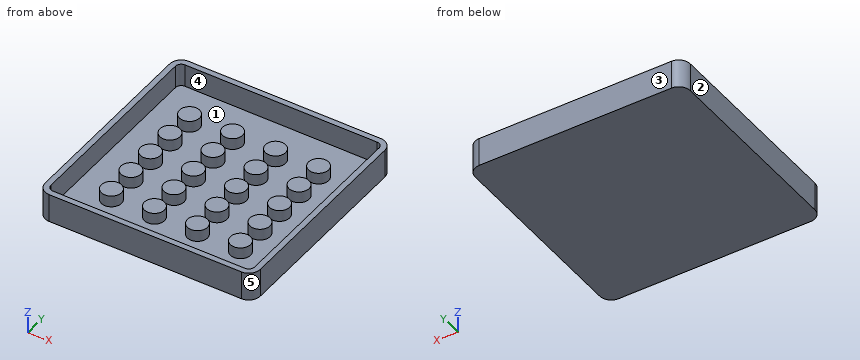
```python
from build123d import *

# Parameters (mm, degrees)
SKETCH1_W           = 75
SKETCH1_H           = 75
BOSS_EXTRUDE1_DEPTH = 10
FILLET1_R           = 4
SHELL1_T            = -2
SKETCH2_R           = 3.5
BOSS_EXTRUDE2_DEPTH = 4


with BuildPart() as part:
    # Sketch1 → Boss-Extrude1 (new body)
    with BuildSketch(Plane.XY):
        with Locations((37.5, 37.5)):
            Rectangle(SKETCH1_W, SKETCH1_H)
    extrude(amount=BOSS_EXTRUDE1_DEPTH)

    # Fillet1
    fillet1_edges = [part.edges().sort_by_distance(p)[0] for p in [
        (0, 75, 5),
        (75, 75, 5),
        (75, 0, 5),
        (0, 0, 5),
    ]]
    fillet(fillet1_edges, radius=FILLET1_R)

    # Shell1
    shell1_openings = [part.faces().sort_by_distance(p)[0] for p in [
        (37.5, 37.5, 10),
    ]]
    offset(amount=SHELL1_T, openings=shell1_openings, kind=Kind.INTERSECTION)

    # Sketch2 → Boss-Extrude2 (add)
    with BuildSketch(Plane.XY.offset(2)):
        with Locations(Location((15, 58.5, 0), (0, 0, 180))):
            Circle(SKETCH2_R)
        with Locations(Location((30, 58.5, 0), (0, 0, 180))):
            Circle(SKETCH2_R)
        with Locations(Location((45, 58.5, 0), (0, 0, 180))):
            Circle(SKETCH2_R)
        with Locations(Location((60, 58.5, 0), (0, 0, 180))):
            Circle(SKETCH2_R)
        with Locations(Location((30, 48, 0), (0, 0, 180))):
            Circle(SKETCH2_R)
        with Locations(Location((45, 48, 0), (0, 0, 180))):
            Circle(SKETCH2_R)
        with Locations(Location((60, 48, 0), (0, 0, 180))):
            Circle(SKETCH2_R)
        with Locations(Location((30, 37.5, 0), (0, 0, 180))):
            Circle(SKETCH2_R)
        with Locations(Location((45, 37.5, 0), (0, 0, 180))):
            Circle(SKETCH2_R)
        with Locations(Location((60, 37.5, 0), (0, 0, 180))):
            Circle(SKETCH2_R)
        with Locations(Location((30, 27, 0), (0, 0, 180))):
            Circle(SKETCH2_R)
        with Locations(Location((45, 27, 0), (0, 0, 180))):
            Circle(SKETCH2_R)
        with Locations(Location((60, 27, 0), (0, 0, 180))):
            Circle(SKETCH2_R)
        with Locations(Location((30, 16.5, 0), (0, 0, 180))):
            Circle(SKETCH2_R)
        with Locations(Location((45, 16.5, 0), (0, 0, 180))):
            Circle(SKETCH2_R)
        with Locations(Location((60, 16.5, 0), (0, 0, 180))):
            Circle(SKETCH2_R)
        with Locations(Location((15, 48, 0), (0, 0, 180))):
            Circle(SKETCH2_R)
        with Locations(Location((15, 37.5, 0), (0, 0, 180))):
            Circle(SKETCH2_R)
        with Locations(Location((15, 27, 0), (0, 0, 180))):
            Circle(SKETCH2_R)
        with Locations(Location((15, 16.5, 0), (0, 0, 180))):
            Circle(SKETCH2_R)
    extrude(amount=BOSS_EXTRUDE2_DEPTH)


solid = part.part
```
Part model, mm, in its own coordinate system. Face numbers are marked on the shaded views. A direction names the side the tool comes from. Round coordinates to 2 decimals unless told otherwise and drop trailing zeros. Write each loop counter-clockwise with the first axis right and the second up, starting at its lowest first coordinate (ties: lowest second). Pieces come first, ordered by that corner, then holes. Notation, with made-up numbers: M 14.5,-22.75 L 69.5,-22.75 A17 ccw 69.5,3.25 Z; hole C 80,74 d8. An arc over 180 degrees is marked long. One line per question, with ' | ' between items.
(1) Probe line 1 along Y through (x, z) = (52, 8.5); line 2 along X through (y, z) = (28, 2.5). List the from-to ranges inside material, lowest first.
Answer key:
line 1: y = 0 to 2, 73 to 75 | line 2: x = 0 to 2, 11.65 to 18.35, 26.65 to 33.35, 41.65 to 48.35, 56.65 to 63.35, 73 to 75
(2) Saw through at B-B on z = 7.25. Write the cut outline in (x, y).
Answer key:
outline: M 0,4 A4 ccw 4,0 L 71,0 A4 ccw 75,4 L 75,71 A4 ccw 71,75 L 4,75 A4 ccw 0,71 Z; hole M 2,4 A2 ccw 4,2 L 71,2 A2 ccw 73,4 L 73,71 A2 ccw 71,73 L 4,73 A2 ccw 2,71 Z
(3) Saw through at A-A on x = 30. Write the cut outline in (y, z).
Answer key:
outline: M 0,0 L 75,0 L 75,10 L 73,10 L 73,2 L 62,2 L 62,6 L 55,6 L 55,2 L 51.5,2 L 51.5,6 L 44.5,6 L 44.5,2 L 41,2 L 41,6 L 34,6 L 34,2 L 30.5,2 L 30.5,6 L 23.5,6 L 23.5,2 L 20,2 L 20,6 L 13,6 L 13,2 L 2,2 L 2,10 L 0,10 Z
(4) 3-axis set-ups, long thin cutter, end or side, ignore diameter. For the marked faces 1 and 2: which of +Z, -Z, +X, -X, +Y, -Y reach the whole face in a straight line?
Answer key:
face 1: +Z | face 2: +Z, -Z, -X, +Y, -Y
(5) Saw through at D-D on y = 48. Write the cut outline in (x, z).
Answer key:
outline: M 0,0 L 75,0 L 75,10 L 73,10 L 73,2 L 63.5,2 L 63.5,6 L 56.5,6 L 56.5,2 L 48.5,2 L 48.5,6 L 41.5,6 L 41.5,2 L 33.5,2 L 33.5,6 L 26.5,6 L 26.5,2 L 18.5,2 L 18.5,6 L 11.5,6 L 11.5,2 L 2,2 L 2,10 L 0,10 Z
(6) Two-plate mould, pull along X, no slides. Class the marked faces 3, 4 and 5: released by +X, released by -X, zero draft, split by the parting line, or undercut.
Answer key:
face 3: zero draft | face 4: undercut | face 5: released by +X
(7) Saw through at C-C on y = 5. Write the cut outline in (x, z).
Answer key:
outline: M 0,0 L 75,0 L 75,10 L 73,10 L 73,2 L 2,2 L 2,10 L 0,10 Z
(8) Pin check, flat tips, straight feed: pin 1 (5.5 mm diameter, centred on x = 45.5, y = 17.5, fed in from +Z); pin 2 (5 mm diameter, centred on x = 64, y = 26.5, fed in from -Z). Stop position of each tip, or through.
Answer key:
pin 1: stops at z = 6 | pin 2: stops at z = 0
